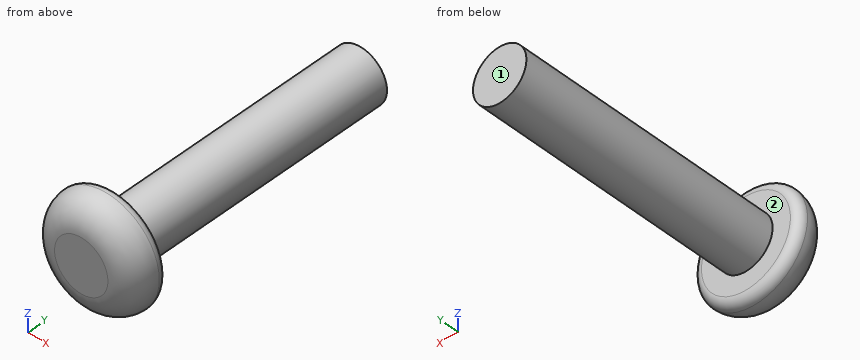
from build123d import *

# Parameters (mm, degrees)
F0_R     = 1.5
F1_DEPTH = 15
F2_R     = 3
F3_DEPTH = 2
F4_R     = 1.5
F5_R     = 0.49999


# Not quite as in the source:
# - a fillet or chamfer is up to 0.001 mm smaller than in the source, because OpenCascade refuses the exact size


with BuildPart() as f1:
    # F0 (on Front) → F1 (new body)
    with BuildSketch(Plane.XZ):
        Circle(F0_R)
    extrude(amount=-F1_DEPTH)

    # F2 (on face) → F3 (join)
    with BuildSketch(Plane.XZ):
        Circle(F2_R)
    extrude(amount=F3_DEPTH)

    # F4
    f4_edges = [f1.edges().sort_by_distance(p)[0] for p in [
        (-3, -2, 0),
    ]]
    fillet(f4_edges, radius=F4_R)

    # F5 (radius 0.5 in the source; OpenCascade refuses exactly that, so slightly less here)
    f5_edges = [f1.edges().sort_by_distance(p)[0] for p in [
        (-3, 0, 0),
    ]]
    fillet(f5_edges, radius=F5_R)


solid = f1.part
Verification items for the finished model (mm, model axes). Face numbers are marked on the shaded views. A direction names the side the tool comes from. Coordinates: 2 decimals unless noted, no trailing zeros. Loops run counter-clockwise (first coordinate to the right, second up) from the corner with the lowest first, then second, coordinate; pieces in that order, holes last. Notation, with made-up numbers: (47, 69.5) -> (51, 69.5) arc R19 ccw to (51, 76.5) -> close; hole circle Ø1 at (2.5, 77.25). An arc over 180 degrees is marked (long way). Answer as CSV lines item,"result".
1) Cross-section at A-A, the plane y = 6.25. Record the cut outline in (x, z), then the cut area to 3 significant figures.
Found:
outline,"circle Ø3 at (0, 0)"
area,"7.07 mm2"
2) Depth check by flat-ended pin: pin 1 (1 mm diameter, centred on x = 2, z = 1.5, fed in from -Y); pin 2 (1.5 mm diameter, centred on y = 10.5, z = -1.5, fed in from +X); pin 3 (1 mm diameter, centred on y = 3, z = 0, fed in from +X). Enter the tip coordinate at first touch or a pass-through.
Found:
pin 1,"stops at y = -1.91"
pin 2,"stops at x = 1.3"
pin 3,"stops at x = 1.5"
3) Tool access check on the marked faces 1 and 2. Record the directions out of +Z, -Z, +X, -X, +Y, -Y that give a thin tool (end or side, any length) a straight path to the whole face; none if there is none.
Found:
face 1,"+Z, -Z, +X, -X, +Y"
face 2,"+Y"
4) Thickness scan on L1, parallel to Y at x = -0.4, z = -1.5; L2, parallel to Z at x = 0.7, y = 5.25; L3, parallel to Z at x = -1.7, y = -0.5. Record the ranges inside material, lowest first. Write a range as from..to.
Found:
L1,"y = -2..0"
L2,"z = -1.33..1.33"
L3,"z = -2.47..2.47"
